Input: part model. Units: mm. Frame: model coordinates. Give positions to 0.01 mm unless a question says otherwise; leave off trailing zeros. Loops run counter-clockwise (first coordinate to the right, second up) from the corner with the lowest first, then second, coordinate; pieces in that order, holes last. Notation, with made-up numbers: (81, 21) - (116, 21) arc R33 cw to (116, 49) - close; hole circle Ø11 at (61.5, 21.25). An arc over 180 degrees is marked (long way). Answer as a JSON object with one key per item and string values. Group by question number.
(1) Section query B-B (z = -22.6). Return loops of the section in (x, y).
(2) Section query C-C (z = -1.5). Return loops of the section in (x, y).
(3) Pin query (flat end, axial travel): P1, Ø8, axis at x = 18.5, z = 24, coming from the +Y side; P2, Ø2.5, axis at x = -10, z = -22.6, coming from the -Y side; P3, Ø6.5, axis at x = -19, z = -21.5, coming from the +Y side; P4, Ø1.2, axis at x = -10.5, y = -2, coming from the -Z side. Return the tip coordinate at first contact, or that it passes through.
(4) Section query A-A (x = 4). Return loops of the section in (y, z), plus the area to 3 significant figures.
(5) Material intervals for L1, parallel to Z at x = -19, y = -3.75; L2, parallel to X at y = -7.25, z = 4; L3, parallel to X at y = -2.75, z = -29, sorted ascending.
```python
from build123d import *

# Parameters (mm, degrees)
F0_W      = 65
F0_H      = 65
F1_DEPTH  = 15
F3_DEPTH  = 15
F5_DEPTH  = 25
F6_R      = 5
F7_DEPTH  = 11
F8_R      = 2
F9_DEPTH  = 25
F10_R     = 5
F11_DEPTH = 11
F13_DEPTH = 4
F14_R     = 4
F15_DEPTH = 6
F16_DEPTH = 7


# Not quite as in the source:
# - the program builds the solid bodies; features that only make, move or delete a surface that nothing else refers to are left out


with BuildPart() as f1:
    # F0 (on Front) → F1 (new body)
    with BuildSketch(Plane.XZ):
        Rectangle(F0_W, F0_H)
    extrude(amount=F1_DEPTH)

    # F2 (on face) → F3 (cut)
    with BuildSketch(Plane.XZ.offset(15)):
        with BuildLine():
            ThreePointArc((18.25, 3.4), (-12.9046987567, 16.3046987567), (0, -14.85))
            ThreePointArc((0, -14.85), (12.9046987567, -9.5046987567), (18.25, 3.4))
        make_face()
    extrude(amount=-F3_DEPTH, mode=Mode.SUBTRACT)

    # F4 (on face) → F5 (cut)
    with BuildSketch(Plane.XZ.offset(15)):
        with BuildLine():
            ThreePointArc((-20.0981694395, 20.6717568643), (-19.4320900923, 21.4178765299), (-18.7383297014, 22.1383297014))
            Line((-18.7383297014, 22.1383297014), (-20.1525432638, 23.5525432638))
            ThreePointArc((-20.1525432638, 23.5525432638), (-20.7379735443, 22.1005871312), (-20.0981694395, 20.6717568643))
        make_face()
        with BuildLine():
            ThreePointArc((18.7383297014, 22.1383297014), (19.4320900923, 21.4178765299), (20.0981694395, 20.6717568643))
            ThreePointArc((20.0981694395, 20.6717568643), (20.5713162639, 21.338229544), (20.7383297014, 22.1383297014))
            ThreePointArc((20.7383297014, 22.1383297014), (20.5860887665, 22.9036965662), (20.1525432638, 23.5525432638))
            Line((20.1525432638, 23.5525432638), (18.7383297014, 22.1383297014))
        make_face()
        with BuildLine():
            Line((17.3241161391, 20.7241161391), (18.7383297014, 22.1383297014))
            ThreePointArc((18.7383297014, 22.1383297014), (18.0178765299, 22.8320900923), (17.2717568643, 23.4981694395))
            ThreePointArc((17.2717568643, 23.4981694395), (16.7386858586, 22.1005871312), (17.3241161391, 20.7241161391))
        make_face()
        with BuildLine():
            ThreePointArc((17.2717568643, 23.4981694395), (18.0178765299, 22.8320900923), (18.7383297014, 22.1383297014))
            Line((18.7383297014, 22.1383297014), (20.1525432638, 23.5525432638))
            ThreePointArc((20.1525432638, 23.5525432638), (18.7005871312, 24.1379735443), (17.2717568643, 23.4981694395))
        make_face()
        with BuildLine():
            ThreePointArc((17.3241161391, 20.7241161391), (18.7005871312, 20.1386858586), (20.0981694395, 20.6717568643))
            ThreePointArc((20.0981694395, 20.6717568643), (19.4320900923, 21.4178765299), (18.7383297014, 22.1383297014))
            Line((18.7383297014, 22.1383297014), (17.3241161391, 20.7241161391))
        make_face()
        with BuildLine():
            ThreePointArc((20.7383297014, -15.3383297014), (20.5713162639, -14.538229544), (20.0981694395, -13.8717568643))
            ThreePointArc((20.0981694395, -13.8717568643), (19.4320900923, -14.6178765299), (18.7383297014, -15.3383297014))
            Line((18.7383297014, -15.3383297014), (20.1525432638, -16.7525432638))
            ThreePointArc((20.1525432638, -16.7525432638), (20.5860887665, -16.1036965662), (20.7383297014, -15.3383297014))
        make_face()
        with BuildLine():
            ThreePointArc((18.7383297014, -15.3383297014), (19.4320900923, -14.6178765299), (20.0981694395, -13.8717568643))
            ThreePointArc((20.0981694395, -13.8717568643), (18.7005871312, -13.3386858586), (17.3241161391, -13.9241161391))
            Line((17.3241161391, -13.9241161391), (18.7383297014, -15.3383297014))
        make_face()
        with BuildLine():
            Line((20.1525432638, -16.7525432638), (18.7383297014, -15.3383297014))
            ThreePointArc((18.7383297014, -15.3383297014), (18.0178765299, -16.0320900923), (17.2717568643, -16.6981694395))
            ThreePointArc((17.2717568643, -16.6981694395), (18.7005871312, -17.3379735443), (20.1525432638, -16.7525432638))
        make_face()
        with BuildLine():
            ThreePointArc((17.2717568643, -16.6981694395), (18.0178765299, -16.0320900923), (18.7383297014, -15.3383297014))
            Line((18.7383297014, -15.3383297014), (17.3241161391, -13.9241161391))
            ThreePointArc((17.3241161391, -13.9241161391), (16.7386858586, -15.3005871312), (17.2717568643, -16.6981694395))
        make_face()
        with BuildLine():
            ThreePointArc((-18.7383297014, 22.1383297014), (-18.0178765299, 22.8320900923), (-17.2717568643, 23.4981694395))
            ThreePointArc((-17.2717568643, 23.4981694395), (-18.7005871312, 24.1379735443), (-20.1525432638, 23.5525432638))
            Line((-20.1525432638, 23.5525432638), (-18.7383297014, 22.1383297014))
        make_face()
        with BuildLine():
            ThreePointArc((-16.7383297014, 22.1383297014), (-16.8764562264, 22.8686906826), (-17.2717568643, 23.4981694395))
            ThreePointArc((-17.2717568643, 23.4981694395), (-18.0178765299, 22.8320900923), (-18.7383297014, 22.1383297014))
            Line((-18.7383297014, 22.1383297014), (-17.3241161391, 20.7241161391))
            ThreePointArc((-17.3241161391, 20.7241161391), (-16.8905706364, 21.3729628367), (-16.7383297014, 22.1383297014))
        make_face()
        with BuildLine():
            Line((-17.3241161391, 20.7241161391), (-18.7383297014, 22.1383297014))
            ThreePointArc((-18.7383297014, 22.1383297014), (-19.4320900923, 21.4178765299), (-20.0981694395, 20.6717568643))
            ThreePointArc((-20.0981694395, 20.6717568643), (-18.7005871312, 20.1386858586), (-17.3241161391, 20.7241161391))
        make_face()
        with BuildLine():
            ThreePointArc((-18.7383297014, -15.3383297014), (-18.0178765299, -16.0320900923), (-17.2717568643, -16.6981694395))
            ThreePointArc((-17.2717568643, -16.6981694395), (-16.8764562264, -16.0686906826), (-16.7383297014, -15.3383297014))
            ThreePointArc((-16.7383297014, -15.3383297014), (-16.8905706364, -14.5729628367), (-17.3241161391, -13.9241161391))
            Line((-17.3241161391, -13.9241161391), (-18.7383297014, -15.3383297014))
        make_face()
        with BuildLine():
            Line((-20.1525432638, -16.7525432638), (-18.7383297014, -15.3383297014))
            ThreePointArc((-18.7383297014, -15.3383297014), (-19.4320900923, -14.6178765299), (-20.0981694395, -13.8717568643))
            ThreePointArc((-20.0981694395, -13.8717568643), (-20.7379735443, -15.3005871312), (-20.1525432638, -16.7525432638))
        make_face()
        with BuildLine():
            ThreePointArc((-20.1525432638, -16.7525432638), (-18.7005871312, -17.3379735443), (-17.2717568643, -16.6981694395))
            ThreePointArc((-17.2717568643, -16.6981694395), (-18.0178765299, -16.0320900923), (-18.7383297014, -15.3383297014))
            Line((-18.7383297014, -15.3383297014), (-20.1525432638, -16.7525432638))
        make_face()
        with BuildLine():
            ThreePointArc((-20.0981694395, -13.8717568643), (-19.4320900923, -14.6178765299), (-18.7383297014, -15.3383297014))
            Line((-18.7383297014, -15.3383297014), (-17.3241161391, -13.9241161391))
            ThreePointArc((-17.3241161391, -13.9241161391), (-18.7005871312, -13.3386858586), (-20.0981694395, -13.8717568643))
        make_face()
    extrude(amount=-F5_DEPTH, mode=Mode.SUBTRACT)

    # F6 (on face) → F7 (cut)
    with BuildSketch(Plane(origin=(0, 0, 0), x_dir=(-1, 0, 0), z_dir=(0, 1, 0))):
        with Locations((-18.7383297014, 22.1383297014)):
            Circle(F6_R)
        with Locations((18.7383297014, 22.1383297014)):
            Circle(F6_R)
        with Locations((-18.7383297014, -15.3383297014)):
            Circle(F6_R)
        with Locations((18.7383297014, -15.3383297014)):
            Circle(F6_R)
    extrude(amount=-F7_DEPTH, mode=Mode.SUBTRACT)

    # F8 (on face) → F9 (cut)
    with BuildSketch(Plane(origin=(0, 0, 0), x_dir=(-1, 0, 0), z_dir=(0, 1, 0))):
        with BuildLine():
            ThreePointArc((12, -22.6), (10, -20.6), (8, -22.6))
            ThreePointArc((8, -22.6), (10, -24.6), (12, -22.6))
        make_face()
        with Locations((-10, -22.6)):
            Circle(F8_R)
    extrude(amount=-F9_DEPTH, mode=Mode.SUBTRACT)

    # F10 (on face) → F11 (cut)
    with BuildSketch(Plane.XZ.offset(15)):
        with Locations((-10, -22.6)):
            Circle(F10_R)
        with Locations((10, -22.6)):
            Circle(F10_R)
    extrude(amount=-F11_DEPTH, mode=Mode.SUBTRACT)

    # F12 (on face) → F13 (cut)
    with BuildSketch(Plane(origin=(0, 0, -32.5), x_dir=(1, 0, 0), z_dir=(0, 0, -1))):
        with BuildLine():
            ThreePointArc((-8, 2.5), (-11.4142135624, 3.9142135624), (-10, 0.5))
            Line((-10, 0.5), (-10, 2.5))
            Line((-10, 2.5), (-8, 2.5))
        make_face()
        with BuildLine():
            ThreePointArc((12, 2.5), (10, 4.5), (8, 2.5))
            ThreePointArc((8, 2.5), (10, 0.5), (12, 2.5))
        make_face()
        with BuildLine():
            Line((-10, 2.5), (-10, 0.5))
            ThreePointArc((-10, 0.5), (-8.5857864376, 1.0857864376), (-8, 2.5))
            Line((-8, 2.5), (-10, 2.5))
        make_face()
    extrude(amount=-F13_DEPTH, mode=Mode.SUBTRACT)

    # F14 (on face) → F15 (cut)
    with BuildSketch(Plane(origin=(0, 0, 0), x_dir=(-1, 0, 0), z_dir=(0, 1, 0))):
        with Locations((-19, -21.5)):
            Circle(F14_R)
        with BuildLine():
            ThreePointArc((23, -21.5), (19, -17.5), (15, -21.5))
            ThreePointArc((15, -21.5), (19, -25.5), (23, -21.5))
        make_face()
    extrude(amount=-F15_DEPTH, mode=Mode.SUBTRACT)

    # F16 (add): a face of the model
    f16_faces = [f1.faces().sort_by_distance(p)[0] for p in [
        (0, -7.5, 32.5),
    ]]
    extrude(f16_faces, amount=F16_DEPTH)


solid = f1.part
```
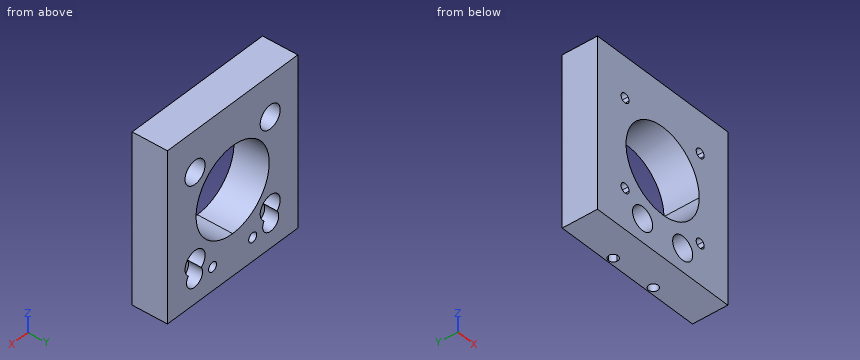
Recorded:
{
 "1": {"outline": "(-32.5, -15) - (-15, -15) - (-15, -4) - (-12, -4) - (-12, 0) - (-15.15, 0) - (-15.15, -6) - (-22.85, -6) - (-22.85, 0) - (-32.5, 0) - close; (-8, -4) - (-5, -4) - (-5, -15) - (5, -15) - (5, -4) - (8, -4) - (8, 0) - (-8, 0) - close; (12, -4) - (15, -4) - (15, -15) - (32.5, -15) - (32.5, 0) - (22.85, 0) - (22.85, -6) - (15.15, -6) - (15.15, 0) - (12, 0) - close"},
 "2": {"outline": "(-32.5, -15) - (-17.58, -15) - (-17.58, 0) - (-32.5, 0) - close; (17.58, -15) - (32.5, -15) - (32.5, 0) - (17.58, 0) - close"},
 "3": {"P1": "stops at y = 0", "P2": "passes through", "P3": "stops at y = -6", "P4": "stops at z = -28.5"},
 "4": {"outline": "(-15, -32.5) - (0, -32.5) - (0, -14.41) - (-15, -14.41) - close; (-15, 21.21) - (0, 21.21) - (0, 39.5) - (-15, 39.5) - close", "area": "546 mm^2"},
 "5": {"L1": "z = -32.5 to -25.5, -10.35 to 17.15, 27.13 to 39.5", "L2": "x = -32.5 to -18.24, 18.24 to 32.5", "L3": "x = -32.5 to -11.98, -8.02 to 8.02, 11.98 to 32.5"}
}
